from build123d import *

# Parameters (mm, degrees)
BOSS_EXTRUDE1_DEPTH = 9.525
SKETCH1_3_W         = 30
SKETCH1_3_H         = 15
SKETCH1_3_R         = 1.5
BOSS_EXTRUDE2_DEPTH = 3.175


with BuildPart() as part:
    # Sketch1 → Boss-Extrude1 (new body)
    with BuildSketch(Plane(origin=(0, 0, 0), x_dir=(1, 0, 0), z_dir=(0, 1, 0))):
        with BuildLine():
            Line((10.4, 7.5), (15, 7.5))
            Line((15, 7.5), (19.6, 7.5))
            ThreePointArc((19.6, 7.5), (15, 12.1), (10.4, 7.5))
        make_face()
        with BuildLine():
            Line((19.6, 7.5), (15, 7.5))
            Line((15, 7.5), (10.4, 7.5))
            ThreePointArc((10.4, 7.5), (15, 2.9), (19.6, 7.5))
        make_face()
    extrude(amount=BOSS_EXTRUDE1_DEPTH)

    # Sketch1_3 → Boss-Extrude2 (add)
    with BuildSketch(Plane(origin=(0, 0, 0), x_dir=(1, 0, 0), z_dir=(0, 1, 0))):
        with Locations((15, 7.5)):
            Rectangle(SKETCH1_3_W, SKETCH1_3_H)
        with Locations(Location((25, 7.5, 0), (0, 0, 270))):
            Circle(SKETCH1_3_R, mode=Mode.SUBTRACT)
        with Locations(Location((5, 7.5, 0), (0, 0, 270))):
            Circle(SKETCH1_3_R, mode=Mode.SUBTRACT)
    extrude(amount=BOSS_EXTRUDE2_DEPTH)


solid = part.part
Work out the finished part from the listing and answer in its coordinate system (mm). Give positions to 0.01 mm unless a question says otherwise; leave off trailing zeros. Order: outer loops, then holes, each group sorted by start corner. A loop starts at its lowest first (then second) coordinate and runs counter-clockwise, first axis right, second up. Notation, with made-up numbers: M 41,44.25 L 89,44.25 A8 ccw 89,57.25 Z; hole C 79,-39.75 d5. An arc over 180 degrees is marked long. Return JSON: item names as keys, results as strings.
Q1. The mould has two halves that part along X. Classify faces 1 (the face through (0, 2, -7)), 2 (the face through (19.596, 6.306, -7.298)), 3 (the face through (26.487, 1.565, -7.695)), 4 (the face through (15, 9.525, -8)): pulls with the +X half, pulls with the -X half, needs draft (parallel to the pull), parting line crosses it, or undercut.
Answer below:
{"face 1": "pulls with the -X half", "face 2": "parting line crosses it", "face 3": "undercut", "face 4": "needs draft"}
Q2. Each of these flat-tipped pins is pushed along its axis until it touches: pin 1 (2.5 mm diameter, centred on x = 5, z = -7.5, fed in from -Y); pin 2 (3 mm diameter, centred on y = 7, z = -3, fed in from -X); pin 3 (3.5 mm diameter, centred on x = 25, z = -7.5, fed in from +Y) (3 decimals). Where does it stop, or does it pass through?
Answer below:
{"pin 1": "passes through", "pin 2": "stops at x = 11.51", "pin 3": "stops at y = 3.175"}
Q3. Find the intervals of material crossed by line 1 along X through (y, z) = (1.7, -7.5); line 2 along X through (y, z) = (1.5, -8.25); line 3 along Y through (x, z) = (9.75, -14) (3 decimals), in increasing order. Write a range as [from, to].
Answer below:
{"line 1": "x = [0, 3.5], [6.5, 23.5], [26.5, 30]", "line 2": "x = [0, 3.7], [6.3, 23.7], [26.3, 30]", "line 3": "y = [0, 3.175]"}
Q4. Find section B-B, the plane y = 1. Write down the section's boundary in (x, z).
Answer below:
{"outline": "M 0,-15 L 30,-15 L 30,0 L 0,0 Z; hole C 5,-7.5 d3; hole C 25,-7.5 d3"}
Q5. Find section D-D, the plane x = 15. Write down the section's boundary in (y, z) (3 decimals), and give its area (3 significant figures).
Answer below:
{"outline": "M 0,-15 L 3.175,-15 L 3.175,-12.1 L 9.525,-12.1 L 9.525,-2.9 L 3.175,-2.9 L 3.175,0 L 0,0 Z", "area": "106 mm^2"}
Q6. Find section C-C, the plane z = -8.5. Write down the section's boundary in (x, y) (3 decimals).
Answer below:
{"outline": "M 0,0 L 3.882,0 L 3.882,3.175 L 0,3.175 Z; M 6.118,0 L 23.882,0 L 23.882,3.175 L 19.49,3.175 L 19.49,9.525 L 10.51,9.525 L 10.51,3.175 L 6.118,3.175 Z; M 26.118,0 L 30,0 L 30,3.175 L 26.118,3.175 Z"}
Q7. Find section A-A, the plane x = 25. Write down the section's boundary in (y, z) (3 decimals).
Answer below:
{"outline": "M 0,-15 L 3.175,-15 L 3.175,-9 L 0,-9 Z; M 0,-6 L 3.175,-6 L 3.175,0 L 0,0 Z"}
